Here's how the part is built. I have some questions about the finished solid (model axes, mm). A direction names the side the tool comes from. Round coordinates to 2 decimals unless told otherwise and drop trailing zeros. Order: outer loops, then holes, each group sorted by start corner. A loop starts at its lowest first (then second) coordinate and runs counter-clockwise, first axis right, second up. Notation, with made-up numbers: M -31,13.25 L -19,13.25 A36 cw -19,48.25 Z; hole C 15,88.5 d10. An arc over 180 degrees is marked long. Write item = value, one per line. Start each with the question number.
Item 1: I want a section at B-B, the plane y = 1. List the corners of the cut face in (x, z) for me, plus the area to 3 significant figures.
Item 2: Please list where these lines run through material, in increasing order: L1, parallel to Y at x = 0, z = 3.7; L2, parallel to Z at x = -2, y = 2.5; L3, parallel to X at y = 10.5, z = 0.25.
Item 3: We'd pull the mould along Z, two halves only. Please class faces 1 (the face through (0, 18, 3)), 2 (the face through (-2.3, 8.87, 5.54)), 3 (the face through (0.1, 9.1, -2.5)): pulls with the +Z half, pulls with the -Z half, needs draft (parallel to the pull), parting line crosses it, or undercut.
Item 4: I want a section at A-A, the plane z = 0. List the corners of the cut face in (x, y) for me (3 decimals).
Item 5: I'm going to push flat-ended pins straight in: P1, Ø2, axis at x = 4.5, y = 15.5, coming from the -Z side; P2, Ø6, axis at x = 0, z = 0, coming from the -Y side (3 decimals); P3, Ø5, axis at x = 3, y = 3, coming from the +Z side. Where does each tip first touch, or does it pass through?
Item 6: I want a section at D-D, the plane y = 15. List the corners of the cut face in (x, z) for me (3 decimals).
Item 7: For faces 4 (the face through (0.672, 16.054, 4.271)), 5 (the face through (-3, 0, 3)), 6 (the face through (1.525, 14.966, 2.302)), which set-ups out of +Z, -Z, +X, -X, +Y, -Y let a thin tool reach every point of the face, with its end or its side?
Item 8: I want a section at C-C, the plane x = -0.5. State how many separate pieces and enclosed holes the cut face has, plus the area to 3 significant figures.
```python
from build123d import *

# Parameters (mm, degrees)
SKETCH1_R                   = 6
SKETCH1_R_2                 = 2.5
BOSS_EXTRUDE1_DEPTH         = 18
M6_TAPPED_HOLE1_D           = 5
M6_TAPPED_HOLE1_DEPTH       = 10
M6_TAPPED_HOLE1_CSINK_D     = 6.05
M6_TAPPED_HOLE1_CSINK_ANGLE = 90
M6_TAPPED_HOLE1_TIP         = 1.502151548


# Read off the part's stored shape, not the designer's step: M3 Tapped Hole1
with BuildPart() as part:
    # Sketch1 → Boss-Extrude1 (new body)
    with BuildSketch(Plane(origin=(0, 0, 0), x_dir=(1, 0, 0), z_dir=(0, 1, 0))):
        with Locations(Location((0, 0, 0), (0, 0, 270))):
            Circle(SKETCH1_R)
        with Locations(Location((0, 0, 0), (0, 0, 270))):
            Circle(SKETCH1_R_2, mode=Mode.SUBTRACT)
    extrude(amount=BOSS_EXTRUDE1_DEPTH)

    # M3 Tapped Hole1 outline → M3 Tapped Hole1 (revolve, cut)
    with BuildSketch(Plane.XZ.offset(-15)):
        Polygon((1.25, 6.000000084), (1.25, 5.725), (1.525000084, 6.000000084), align=None)
        Polygon((1.25, 2.775), (1.25, 5.725), (1.25, 6.000000084), (0, 6.000000084), (0, 1.980737508), (1.25, 1.980737508), align=None)
        Polygon((1.525, 2.5), (1.25, 2.775), (1.25, 1.980737508), (1.525000084, 1.980737508), align=None)
    revolve(axis=Axis((0, 15, 0), (0, 0, 1)), mode=Mode.SUBTRACT)

    # M6 Tapped Hole1
    with Locations(Plane.XZ):
        with Locations((0, 0)):
            CounterSinkHole(M6_TAPPED_HOLE1_D / 2, M6_TAPPED_HOLE1_CSINK_D / 2, depth=M6_TAPPED_HOLE1_DEPTH, counter_sink_angle=M6_TAPPED_HOLE1_CSINK_ANGLE)
            with Locations((0, 0, -(M6_TAPPED_HOLE1_DEPTH + M6_TAPPED_HOLE1_TIP / 2))):  # 118° drill point
                Cone(0, M6_TAPPED_HOLE1_D / 2, M6_TAPPED_HOLE1_TIP, mode=Mode.SUBTRACT)


solid = part.part
```
Filled in:
q1.outline = C 0,0 d12; hole C 0,0 d5
q1.area = 93.5 mm^2
q2.L1 = 0 to 13.75, 16.25 to 18
q2.L2 = -5.66 to -1.5, 1.5 to 5.66
q2.L3 = -5.99 to -2.49, 2.49 to 5.99
q3.face_1 = needs draft
q3.face_2 = parting line crosses it
q3.face_3 = undercut
q4.outline = M -6,0 L -3.025,0 L -2.5,0.525 L -2.5,18 L -6,18 Z; M 2.5,0.525 L 3.025,0 L 6,0 L 6,18 L 2.5,18 Z
q5.P1 = -4.87
q5.P2 = 0.025
q5.P3 = 5.98
q6.outline = M -1.525,1.981 L -1.525,2.5 L -1.25,2.775 L -1.25,5.725 L -1.367,5.842 A6 ccw long 1.367,5.842 L 1.25,5.725 L 1.25,2.775 L 1.525,2.5 L 1.525,1.981 A2.5 cw long Z
q7.face_4 = +Z
q7.face_5 = +Z, -Z, +X, -X, -Y
q7.face_6 = none
q8.separate_pieces = 3
q8.enclosed_holes = 0
q8.area = 119 mm^2
